from build123d import *

# Parameters (mm, degrees)
TOP_BLADE_FIRST_EXTRUDE_DEPTH  = 10
SKETCH3_W                      = 40
SKETCH3_H                      = 10
TOP_BLADE_SECOND_EXTRUDE_DEPTH = 1
TOP_BLADE_CUT_1_SIZE           = 1
TOP_BLADE_ROUNDING_1_R         = 1
SKETCH5_R                      = 1
TOP_BLADE_CUT_2_DEPTH          = 19
TOP_BLADE_ROUNDING_2_R         = 1


with BuildPart() as part:
    # Sketch1 → Top Blade First Extrude (new body)
    with BuildSketch(Plane(origin=(0, 0, 0), x_dir=(0, 0, -1), z_dir=(1, 0, 0))):
        Polygon((-14.254658385, 0), (15.745341615, 0), (33.065849691, 10), (32.565849691, 10.866025404), (15.477392422, 1), (-13.840444823, 1), (-34.76075504, 21.920310217), (-35.467861821, 21.213203436), align=None)
    extrude(amount=TOP_BLADE_FIRST_EXTRUDE_DEPTH)

    # Sketch3 → Top Blade Second Extrude (add)
    with BuildSketch(Plane.XZ):
        with Locations((-20, -0.745341615)):
            Rectangle(SKETCH3_W, SKETCH3_H)
        with Locations((30, -0.745341615)):
            Rectangle(SKETCH3_W, SKETCH3_H)
    extrude(amount=-TOP_BLADE_SECOND_EXTRUDE_DEPTH)

    # Top Blade Cut 1
    top_blade_cut_1_edges = [part.edges().sort_by_distance(p)[0] for p in [
        (-20, 1, 4.254658385),
        (0, 5.933012702, -24.021621057),
        (30, 1, -5.745341615),
        (10, 11.460155108, 24.300599931),
    ]]
    chamfer(top_blade_cut_1_edges, length=TOP_BLADE_CUT_1_SIZE - 0.0001)  # a hair under: the kernel refuses the full size

    # Top Blade Rounding 1
    top_blade_rounding_1_edges = [part.edges().sort_by_distance(p)[0] for p in [
        (-40, 0.50005, 3.754708385),
        (50, 0.50005, -5.245391615),
    ]]
    fillet(top_blade_rounding_1_edges, radius=TOP_BLADE_ROUNDING_1_R)

    # Sketch5 → Top Blade Cut 2 (cut)
    with BuildSketch(Plane.XZ):
        with Locations(Location((5, -0.745341615, 0), (0, 0, 270))):
            Circle(SKETCH5_R)
    extrude(amount=-TOP_BLADE_CUT_2_DEPTH, mode=Mode.SUBTRACT)

    # Top Blade Rounding 2
    top_blade_rounding_2_edges = [part.edges().sort_by_distance(p)[0] for p in [
        (4.50005, 1, 13.840444823),
        (5.49995, 1, -15.477392422),
    ]]
    fillet(top_blade_rounding_2_edges, radius=TOP_BLADE_ROUNDING_2_R)


solid = part.part
The listing builds one solid part. Answer for the finished solid, in the listing's coordinates (mm). A direction names the side the tool comes from. Coordinates: 2 decimals unless noted, no trailing zeros. Write each loop counter-clockwise with the first axis right and the second up, starting at its lowest first coordinate (ties: lowest second). Pieces come first, ordered by that corner, then holes. Notation, with made-up numbers: M 67.5,-30.5 L 114.5,-30.5 A9 ccw 114.5,-20.5 Z; hole C 39.5,-10.5 d1. An arc over 180 degrees is marked long. Use one line per item in the form item = value.
Item 1: The mould has two halves that part along Z. Classify faces 5 (the face through (5.843, 0.493, -1.283)), 6 (the face through (4.93, 10.755, 25.01)), 7 (the face through (0, 8.6, 21.8)): released by +Z, released by -Z, zero draft, split by the parting line, or undercut.
Model answer:
face_5 = undercut
face_6 = released by +Z
face_7 = zero draft
Item 2: Given P1, Ø8, axis at x = 14.5, y = 4.5, coming from the -Z side; P2, Ø11, axis at y = 4.5, z = -24.5, coming from the -X side; P3, Ø12, axis at y = 6, z = -19, coming from the +X side, each flat-ended and moving along its own axis, determine where each tip first touches the part or whether it passes through.
Model answer:
P1 = -5.25
P2 = 0
P3 = 10
Item 3: For faces 1 (the face through (0.575, 5.577, -24.255)), 2 (the face through (9.49, 10.86, 24.39)), 3 (the face through (4.44, 11.46, 24.3)), 4 (the face through (0, 0.6, -11.2)), determine the directions among +Z, -Z, +X, -X, +Y, -Y from which every point of the face is accessible in a straight line to the end or side of a thin tool.
Model answer:
face_1 = -X, +Y
face_2 = +X, +Y
face_3 = +X, -X, +Y
face_4 = -Z, -X, +Y, -Y
Item 4: Find section A-A, the plane x = 5. Give the vertices of the cut face in (y, z), plus the area to 3 significant figures.
Model answer:
outline = M 0,-15.75 L 10,-33.07 L 10.87,-32.57 L 1.13,-15.71 A1 cw 1,-15.21 L 1,-1.75 L 0,-1.75 Z; M 0,0.25 L 1,0.25 L 1,13.43 A1 cw 1.29,14.13 L 21.92,34.76 L 21.21,35.47 L 0,14.25 Z
area = 77.3 mm2
Item 5: Find the intervals of material crossed by probe 1 along Y at (x, z) = (-19, -5.5); probe 2 along Y at (x, z) = (7.5, 26.5), in increasing order.
Model answer:
probe_1 = 0 to 1
probe_2 = 12.25 to 13.66
Item 6: Find section D-D, the plane z = -7. Give the vertices of the cut face in (x, y).
Model answer:
outline = M 0,0 L 10,0 L 10,1 L 0,1 Z
